from build123d import *

# Parameters (mm, degrees)
SKETCH1_W           = 44.1
SKETCH1_H           = 120
BOSS_EXTRUDE1_DEPTH = 8.8
FILLET1_R           = 6
CUT_EXTRUDE1_DEPTH  = 121
CUT_EXTRUDE2_DEPTH  = 6


with BuildPart() as part:
    # Sketch1 → Boss-Extrude1 (new body)
    with BuildSketch(Plane(origin=(0, 0, 0), x_dir=(1, 0, 0), z_dir=(0, 1, 0))):
        Rectangle(SKETCH1_W, SKETCH1_H)
        with BuildLine():
            Line((-2.5, -25), (-2.5, 25))
            ThreePointArc((-2.5, 25), (0, 27.5), (2.5, 25))
            Line((2.5, 25), (2.5, -25))
            ThreePointArc((2.5, -25), (0, -27.5), (-2.5, -25))
        make_face(mode=Mode.SUBTRACT)
        with BuildLine():
            Line((-2.5, 36.5), (2.5, 36.5))
            ThreePointArc((2.5, 36.5), (5, 34), (2.5, 31.5))
            Line((2.5, 31.5), (-2.5, 31.5))
            ThreePointArc((-2.5, 31.5), (-5, 34), (-2.5, 36.5))
        make_face(mode=Mode.SUBTRACT)
        with BuildLine():
            Line((-2.5, 44.5), (2.5, 44.5))
            ThreePointArc((2.5, 44.5), (5, 42), (2.5, 39.5))
            Line((2.5, 39.5), (-2.5, 39.5))
            ThreePointArc((-2.5, 39.5), (-5, 42), (-2.5, 44.5))
        make_face(mode=Mode.SUBTRACT)
        with BuildLine():
            Line((-2.5, -44.5), (2.5, -44.5))
            ThreePointArc((2.5, -44.5), (5, -42), (2.5, -39.5))
            Line((2.5, -39.5), (-2.5, -39.5))
            ThreePointArc((-2.5, -39.5), (-5, -42), (-2.5, -44.5))
        make_face(mode=Mode.SUBTRACT)
        with BuildLine():
            Line((-2.5, -36.5), (2.5, -36.5))
            ThreePointArc((2.5, -36.5), (5, -34), (2.5, -31.5))
            Line((2.5, -31.5), (-2.5, -31.5))
            ThreePointArc((-2.5, -31.5), (-5, -34), (-2.5, -36.5))
        make_face(mode=Mode.SUBTRACT)
    extrude(amount=BOSS_EXTRUDE1_DEPTH)

    # Fillet1
    fillet1_edges = [part.edges().sort_by_distance(p)[0] for p in [
        (22.05, 4.4, 60),
        (-22.05, 4.4, 60),
        (-22.05, 4.4, -60),
        (22.05, 4.4, -60),
    ]]
    fillet(fillet1_edges, radius=FILLET1_R)

    # Sketch2 → Cut-Extrude1 (cut, through all)
    with BuildSketch(Plane.XY.offset(60)):
        Polygon((19.25, 0), (19.25, 1.270336268), (16.65, 4.958404732), (16.65, 5.1), (22.05, 5.1), (22.05, 0), align=None)
        Polygon((-22.05, 0), (-19.25, 0), (-19.25, 1.270336268), (-16.65, 4.958404732), (-16.65, 5.1), (-22.05, 5.1), align=None)
    extrude(amount=-CUT_EXTRUDE1_DEPTH, mode=Mode.SUBTRACT)

    # Sketch3 → Cut-Extrude2 (cut)
    with BuildSketch(Plane.XZ):
        with BuildLine():
            Line((-8.95, -55), (8.95, -55))
            ThreePointArc((8.95, -55), (12.485533906, -53.535533906), (13.95, -50))
            Line((13.95, -50), (13.95, 50))
            ThreePointArc((13.95, 50), (12.485533906, 53.535533906), (8.95, 55))
            Line((8.95, 55), (-8.95, 55))
            ThreePointArc((-8.95, 55), (-12.485533906, 53.535533906), (-13.95, 50))
            Line((-13.95, 50), (-13.95, -50))
            ThreePointArc((-13.95, -50), (-12.485533906, -53.535533906), (-8.95, -55))
        make_face()
    extrude(amount=-CUT_EXTRUDE2_DEPTH, mode=Mode.SUBTRACT)


solid = part.part
Design review of the part built by this model. Coordinates are the model's own, in mm. A direction names the side the tool comes from. Coordinates: 2 decimals unless noted, no trailing zeros. Loops run counter-clockwise (first coordinate to the right, second up) from the corner with the lowest first, then second, coordinate; pieces in that order, holes last. Notation, with made-up numbers: M -28.75,74 L -23.75,74 A38 cw -23.75,113 Z; hole C -37,78 d10. An arc over 180 degrees is marked long. Answer as CSV lines item,"result".
Item 1: Machinability: for faces 5 (the face through (-0.1, 7.4, -27.5)), 6 (the face through (0, 4, -60)), 7 (the face through (-12.45, 2.96, 53.57)), which of the approach directions +Z, -Z, +X, -X, +Y, -Y give a long, thin tool a straight path to every point of the face, cutting with its end or side? Answer none if there is none.
Answer list:
face 5,"+Y, -Y"
face 6,"-Z, +X, -X, +Y, -Y"
face 7,"-Y"
Item 2: For P1, Ø1, axis at x = -11.5, z = 39.5, coming from the -Y side; P2, Ø0.6, axis at y = 0.5, z = 6, coming from the -X side; P3, Ø1, axis at y = 2, z = -32, coming from the +X side; P4, Ø6, axis at x = 20, z = -4.5, coming from the -Y side, all flat-tipped, find the tip position at first contact; note any pin that passes through.
Answer list:
P1,"y = 6"
P2,"x = -19.25"
P3,"x = 19.09"
P4,"y = 0"
Item 3: Add section B-B on x = 0.5. State the section outline as (y, z) points.
Answer list:
outline,"M 0,-60 L 8.8,-60 L 8.8,-44.5 L 6,-44.5 L 6,-55 L 0,-55 Z; M 0,55 L 6,55 L 6,44.5 L 8.8,44.5 L 8.8,60 L 0,60 Z; M 6,-39.5 L 8.8,-39.5 L 8.8,-36.5 L 6,-36.5 Z; M 6,-31.5 L 8.8,-31.5 L 8.8,-27.45 L 6,-27.45 Z; M 6,27.45 L 8.8,27.45 L 8.8,31.5 L 6,31.5 Z; M 6,36.5 L 8.8,36.5 L 8.8,39.5 L 6,39.5 Z"
Item 4: Add section C-C on y = 3. State the section outline as (x, z) points.
Answer list:
outline,"M -18.03,-59.66 A6 ccw -16.05,-60 L 16.05,-60 A6 ccw 18.03,-59.66 L 18.03,59.66 A6 ccw 16.05,60 L -16.05,60 A6 ccw -18.03,59.66 Z; hole M -13.95,-50 A5 ccw -8.95,-55 L 8.95,-55 A5 ccw 13.95,-50 L 13.95,50 A5 ccw 8.95,55 L -8.95,55 A5 ccw -13.95,50 Z"
Item 5: For probe 1 along Z at (x, y) = (6.5, 3.75); probe 2 along X at (y, z) = (0.5, -30); probe 3 along X at (y, z) = (7.75, 3), list the stretches that pass through material, from the lowest coordinate up.
Answer list:
probe 1,"-60 to -55, 55 to 60"
probe 2,"-19.25 to -13.95, 13.95 to 19.25"
probe 3,"-22.05 to -2.5, 2.5 to 22.05"
Item 6: Add section A-A on z = 2. State the section outline as (x, y) points.
Answer list:
outline,"M -22.05,5.1 L -16.65,5.1 L -16.65,4.96 L -19.25,1.27 L -19.25,0 L -13.95,0 L -13.95,6 L -2.5,6 L -2.5,8.8 L -22.05,8.8 Z; M 2.5,6 L 13.95,6 L 13.95,0 L 19.25,0 L 19.25,1.27 L 16.65,4.96 L 16.65,5.1 L 22.05,5.1 L 22.05,8.8 L 2.5,8.8 Z"
Item 7: The part is to be moulded in two halves that separate along Z. For faces 1 (the face through (0, 3, 55)), 2 (the face through (22.05, 7, 1)), 3 (the face through (-2.5, 7, 0)), 4 (the face through (19.44, 5.44, 58.95)), say which applies: pulls with the +Z half, pulls with the -Z half, needs draft (parallel to the pull), parting line crosses it, or undercut.
Answer list:
face 1,"undercut"
face 2,"needs draft"
face 3,"undercut"
face 4,"pulls with the +Z half"
Item 8: Add section D-D on x = -18. State the section outline as (y, z) points, plus the area to 3 significant figures.
Answer list:
outline,"M 0,-59.67 L 3.04,-59.67 L 3.04,59.67 L 0,59.67 Z; M 5.1,-59.67 L 8.8,-59.67 L 8.8,59.67 L 5.1,59.67 Z"
area,"805 mm²"
